Check sheet for the modelled part. Datum: model origin and axes. Units: mm. A direction names the side the tool comes from. Coordinates: 2 decimals unless noted, no trailing zeros. Order: outer loops, then holes, each group sorted by start corner. A loop starts at its lowest first (then second) coordinate and runs counter-clockwise, first axis right, second up.
1. Gauge pin test, flat ends, axial feed: pin 1 Ø5 at (x, z) = (57.5, 12) entering from -Y; pin 2 Ø5 at (y, z) = (2, 5) entering from +X. Record the tip position at first contact, or that the pin passes through.
2. Thickness scan on line 1 (Z direction, x = 11, y = 14.5); line 2 (Y direction, x = 33, z = 4); line 3 (X direction, y = 4.75, z = 12). Record the ranges inside material, lowest first.
3. Cross-section at C-C (y = 3.75). Enter the section's corners in (x, z), then the cut area to 3 significant figures.
4. Cross-section at D-D (x = 58). Enter the section's corners in (y, z).
5. Set-up check for faces 5 (the flat face through (52, 11.5, 7)), 6 (the flat face through (33, 14, 15)): record each of +Z, -Z, +X, -X, +Y, -Y from which the full face is reachable in a straight line by a thin tool's end or side.
6. Draft check along Z on faces 1 (the flat face through (85, 17, 7)), 2 (the cylindrical face through (9.75, 10.6, 7.55)), 3 (the cylindrical face through (5.155, 10.599, 7.021)), 4 (the cylindrical face through (40.92, 20.9, 0.57)). Enter one of: released by +Z, released by -Z, zero draft, split by the parting line, or undercut.
7. Cross-section at B-B (x = 11). Enter the section's corners in (y, z), then the cut area to 3 significant figures.
8. Cross-section at A-A (z = 7.5). Enter the section's corners in (x, y), then the cut area to 3 significant figures.
```python
from build123d import *

# Parameters (mm, degrees)
BOSS_EXTRUDE1_DEPTH = 15
SKETCH2_R           = 1.25
CUT_EXTRUDE1_DEPTH  = 89.950829114
FILLET1_R           = 5
FILLET2_R           = 2
FILLET3_R           = 2


with BuildPart() as part:
    # Sketch1 → Boss-Extrude1 (new body)
    with BuildSketch(Plane.XY):
        Polygon((0, 0), (0, 21.5), (85, 21.5), (85, 11.5), (15, 11.5), (15, 0), align=None)
    extrude(amount=BOSS_EXTRUDE1_DEPTH)

    # Sketch2 → Cut-Extrude1 (cut, through all)
    with BuildSketch(Plane.XZ):
        with Locations((4, 7.5)):
            Circle(SKETCH2_R)
        with Locations((11, 7.5)):
            Circle(SKETCH2_R)
    extrude(amount=-CUT_EXTRUDE1_DEPTH, mode=Mode.SUBTRACT)

    # Fillet1
    fillet1_edges = [part.edges().sort_by_distance(p)[0] for p in [
        (15, 11.5, 7.5),
    ]]
    fillet(fillet1_edges, radius=FILLET1_R)

    # Fillet2
    fillet2_edges = [part.edges().sort_by_distance(p)[0] for p in [
        (85, 21.5, 7.5),
        (85, 11.5, 7.5),
        (85, 16.5, 15),
        (85, 16.5, 0),
    ]]
    fillet(fillet2_edges, radius=FILLET2_R)

    # Fillet3
    # the kernel refuses this fillet: 2 mm, written as the material it takes off along each edge
    with BuildSketch(Plane(origin=(83, 19.5, 13), x_dir=(0, 0, 1), z_dir=(0, 1, 0))) as fillet3_piece_1_section:
        Polygon((0, 0), (FILLET3_R, 0), (FILLET3_R, FILLET3_R), (0, FILLET3_R), align=None)
    fillet3_piece_1 = extrude(amount=FILLET3_R, mode=Mode.PRIVATE)
    fillet3_piece_1 = fillet3_piece_1 - Plane(origin=(83, 19.5, 13), x_dir=(-0.7071067811865475, 2.0097183471152325e-15, -0.7071067811865475), z_dir=(0, 1, 0)) * Sphere(FILLET3_R, mode=Mode.PRIVATE)
    add(fillet3_piece_1, mode=Mode.SUBTRACT)
    with BuildSketch(Plane(origin=(83, 19.5, 2), x_dir=(0, 1, 0), z_dir=(0, 0, -1))) as fillet3_piece_2_section:
        Polygon((0, 0), (FILLET3_R, 0), (FILLET3_R, FILLET3_R), (0, FILLET3_R), align=None)
    fillet3_piece_2 = extrude(amount=FILLET3_R, mode=Mode.PRIVATE)
    fillet3_piece_2 = fillet3_piece_2 - Plane(origin=(83, 19.5, 2), x_dir=(-0.7071067811865486, -0.7071067811865466, 0), z_dir=(0, 0, -1)) * Sphere(FILLET3_R, mode=Mode.PRIVATE)
    add(fillet3_piece_2, mode=Mode.SUBTRACT)
    with BuildSketch(Plane(origin=(0, 21.5, -5), x_dir=(1, 0, 0), z_dir=(0, 0, 1))) as fillet3_piece_3:
        with BuildLine():
            CenterArc((FILLET3_R, -FILLET3_R), FILLET3_R, 90, 90)
            Line((0, -FILLET3_R), (0, 0))
            Line((0, 0), (FILLET3_R, 0))
        make_face()
    extrude(amount=25, mode=Mode.SUBTRACT)
    with BuildSketch(Plane(origin=(-5, 21.5, 0), x_dir=(0, -1, 0), z_dir=(1, 0, 0)), Plane(origin=(-5, 21.5, 15), x_dir=(0, 0, -1), z_dir=(1, 0, 0))) as fillet3_piece_4:
        with BuildLine():
            CenterArc((FILLET3_R, -FILLET3_R), FILLET3_R, 90, 90)
            Line((0, -FILLET3_R), (0, 0))
            Line((0, 0), (FILLET3_R, 0))
        make_face()
    extrude(amount=88, mode=Mode.SUBTRACT)


solid = part.part
```
Data:
1. pin 1: stops at y = 11.5
1. pin 2: stops at x = 15
2. line 1: z = 0 to 6.25, 8.75 to 15
2. line 2: y = 11.5 to 21.5
2. line 3: x = 0 to 15
3. outline: (0, 0) - (15, 0) - (15, 15) - (0, 15) - close; hole circle Ø2.5 at (4, 7.5); hole circle Ø2.5 at (11, 7.5)
3. area: 215 mm2
4. outline: (11.5, 0) - (19.5, 0) arc R2 ccw to (21.5, 2) - (21.5, 13) arc R2 ccw to (19.5, 15) - (11.5, 15) - close
5. face 5: +Z, -Z, +X, -Y
5. face 6: +Z, +X, -X, +Y, -Y
6. face 1: zero draft
6. face 2: undercut
6. face 3: undercut
6. face 4: released by -Z
7. outline: (0, 0) - (19.5, 0) arc R2 ccw to (21.5, 2) - (21.5, 6.25) - (0, 6.25) - close; (0, 8.75) - (21.5, 8.75) - (21.5, 13) arc R2 ccw to (19.5, 15) - (0, 15) - close
7. area: 267 mm2
8. outline: (0, 0) - (2.75, 0) - (2.75, 21.5) - (2, 21.5) arc R2 ccw to (0, 19.5) - close; (5.25, 0) - (9.75, 0) - (9.75, 21.5) - (5.25, 21.5) - close; (12.25, 0) - (15, 0) - (15, 6.5) arc R5 cw to (20, 11.5) - (83, 11.5) arc R2 ccw to (85, 13.5) - (85, 19.5) arc R2 ccw to (83, 21.5) - (12.25, 21.5) - close
8. area: 918 mm2
